```python
from build123d import *

# Parameters (mm, degrees)
SKETCH1_R           = 10.5
BOSS_EXTRUDE1_DEPTH = 76.5
SKETCH3_W           = 3
SKETCH3_H           = 3
BOSS_EXTRUDE2_DEPTH = 12
SKETCH4_R           = 1
BOSS_EXTRUDE3_DEPTH = 2
SKETCH7_R           = 10.5
SKETCH7_W           = 3
SKETCH7_H           = 3
BOSS_EXTRUDE4_DEPTH = 6
BOSS_EXTRUDE5_DEPTH = 159


with BuildPart() as part:
    # Sketch1 → Boss-Extrude1 (new, symmetric)
    with BuildSketch(Plane.XY):
        Circle(SKETCH1_R)
    extrude(amount=BOSS_EXTRUDE1_DEPTH, both=True)

    # Sketch3 → Boss-Extrude2 (add)
    with BuildSketch(Plane(origin=(0, 0, -76.5), x_dir=(-1, 0, 0), z_dir=(0, 0, -1))):
        Rectangle(SKETCH3_W, SKETCH3_H)
    extrude(amount=BOSS_EXTRUDE2_DEPTH)

    # Sketch4 → Boss-Extrude3 (add)
    with BuildSketch(Plane.XY.offset(76.5)):
        Polygon((0, 2.886751346), (-2.5, 1.443375673), (-2.5, -1.443375673), (0, -2.886751346), (2.5, -1.443375673), (2.5, 1.443375673), align=None)
        Circle(SKETCH4_R, mode=Mode.SUBTRACT)
    extrude(amount=BOSS_EXTRUDE3_DEPTH)

    # Sketch7 → Boss-Extrude4 (add)
    with BuildSketch(Plane(origin=(0, 0, -76.5), x_dir=(-1, 0, 0), z_dir=(0, 0, -1))):
        Circle(SKETCH7_R)
        Rectangle(SKETCH7_W, SKETCH7_H, mode=Mode.SUBTRACT)
    extrude(amount=BOSS_EXTRUDE4_DEPTH)

    # Sketch8 → Boss-Extrude5 (add)
    with BuildSketch(Plane.XY.offset(76.5)):
        Polygon((-0.228880958, 10.279411866), (0.985593436, 12.463206486), (2.253499249, 12.295191789), (1.036282986, 10.106466905), align=None)
        Polygon((9.050051597, 8.622445482), (6.778802746, 7.567191623), (5.856918112, 8.450751744), (8.123050808, 9.503628565), align=None)
        Polygon((12.389791835, 1.656218067), (9.93205026, 2.137506341), (9.705573533, 3.394191686), (12.157778863, 2.913987549), align=None)
        Polygon((10.997052705, -5.942628357), (9.291592153, -4.108633713), (9.847029745, -2.958834232), (11.548648621, -4.788697668), align=None)
        Polygon((5.403813218, -11.271592731), (5.102061653, -8.785415336), (6.227255282, -8.18168604), (6.52832713, -10.662263138), align=None)
        Polygon((-2.253499249, -12.295191789), (-1.036282986, -10.106466905), (0.228880958, -10.279411866), (-0.985593436, -12.463206486), align=None)
        Polygon((-9.050051597, -8.622445482), (-6.778802746, -7.567191623), (-5.856918112, -8.450751744), (-8.123050808, -9.503628565), align=None)
        Polygon((-12.389791835, -1.656218067), (-9.93205026, -2.137506341), (-9.705573533, -3.394191686), (-12.157778863, -2.913987549), align=None)
        Polygon((-10.997052705, 5.942628357), (-9.291592153, 4.108633713), (-9.847029745, 2.958834232), (-11.548648621, 4.788697668), align=None)
        Polygon((-5.403813218, 11.271592731), (-5.102061653, 8.785415336), (-6.227255282, 8.18168604), (-6.52832713, 10.662263138), align=None)
    extrude(amount=-BOSS_EXTRUDE5_DEPTH)


solid = part.part
```
Source: CAD feature listing. Evaluate the final solid. Frame: model axes, mm. A direction names the side the tool comes from. Give positions to 0.01 mm unless a question says otherwise; leave off trailing zeros. One line per item, written item: value. Start each with the question number.
Q1. Set-up query: faces 5 (the face through (1.5, 0, -85)), 6 (the face through (0, -1.5, -85)), 7 (the face through (0, 1.5, -85)). Return all of +Z, -Z, +X, -X, +Y, -Y with unobstructed straight access to the full face (end or side cutting, diameter ignored); none if empty.
Q2. Draft query along X for faces 1 (the face through (3, 0, 76.5)), 2 (the face through (-1.5, 0, -85)), 3 (the face through (2.747, -10.134, -1.887)), 4 (the face through (-2.747, 10.134, -1.887)). Return one class per face: +X half, -X half, draft (parallel to the pull), parting line (faces both ways), or undercut.
Q3. First-contact query: pin 1 Ø7.5 at (x, y) = (2.5, 5.5) entering from -Z; pin 2 Ø4 at (x, z) = (5.5, -12.5) entering from +Y; pin 3 Ø6 at (x, z) = (-5.5, 1.5) entering from -Y; pin 4 Ø1.6 at (x, y) = (-0.5, -0.5) entering from +Z. Flat tips, straight axial feed; report the tip coordinate or a pass-through.
Q4. Material intervals for probe 1 along Y at (x, z) = (0, 77.25); probe 2 along Z at (x, y) = (6.5, 3.5); probe 3 along Y at (x, z) = (-4.5, -68), sorted ascending. Write a range as from..to.
Answer:
1. face 5: -Z, +X, +Y, -Y
1. face 6: -Z, +X, -X, -Y
1. face 7: -Z, +X, -X, +Y
2. face 1: draft
2. face 2: -X half
2. face 3: undercut
2. face 4: undercut
3. pin 1: stops at z = -82.5
3. pin 2: stops at y = 9.9
3. pin 3: stops at y = -10.2
3. pin 4: stops at z = 78.5
4. probe 1: y = -2.89..-1, 1..2.89
4. probe 2: z = -82.5..76.5
4. probe 3: y = -9.49..9.49
